The model under review builds one solid part; all positions refer to its coordinate system, in mm. A direction names the side the tool comes from. Round coordinates to 2 decimals unless told otherwise and drop trailing zeros. Write each loop counter-clockwise with the first axis right and the second up, starting at its lowest first coordinate (ties: lowest second). Pieces come first, ordered by that corner, then holes. Notation, with made-up numbers: M 52,72 L 80,72 A9 ccw 80,87 Z; hole C -6,-23.75 d4. An arc over 180 degrees is marked long. Write item = value, one per line. Start each with the question number.
Item 1: Take a section at A-A, the plane x = 0. Give the boundary of the cut face in (y, z) (3 decimals).
Item 2: Tool access review of faces 1 (the cylindrical face through (12.91, 4.83, 15.33)), 2 (the flat face through (-22.225, 5, 2)), 3 (the flat face through (22.225, 5, 2)): name each direction out of +Z, -Z, +X, -X, +Y, -Y from which nothing blocks a thin tool from reaching the whole face with its end or side.
Item 3: For pin 1 Ø25 at (x, z) = (0, 0) entering from +Y; pin 2 Ø3 at (y, z) = (4, -8.5) entering from +X (3 decimals); pin 3 Ø5 at (x, y) = (34.5, 6.5) entering from -Z; pin 4 Ø5 at (y, z) = (4, 9.5) entering from -X (3 decimals), all flat-tipped, find the tip position at first contact; note any pin that passes through.
Item 4: Take a section at B-B, the plane z = 0. Give the boundary of the cut face in (x, y) (3 decimals).
Item 5: To check wall thickness, follow line 1 along X through (y, z) = (3.5, 0) (3 decimals); line 2 along Z through (x, y) = (0, 2.5) (3 decimals); line 3 along Z through (x, y) = (36, 9.25). State the ranges of each line that lie inside material, in increasing order.
Item 6: Take a section at C-C, the plane x = 34. Give the boundary of the cut face in (y, z) (3 decimals), plus the area to 3 significant figures.
Item 7: Take a section at D-D, the plane z = -17.5. Give the boundary of the cut face in (x, y) (3 decimals).
Item 8: The part is to be moulded in two halves that separate along X. For faces 4 (the cylindrical face through (-24.135, 4.829, 29.939)), 5 (the cylindrical face through (8.329, 4.829, -13.065)), 6 (the flat face through (35, 5, 31.75)), say which applies: +X half, -X half, draft (parallel to the pull), parting line (faces both ways), or undercut.
from build123d import *

# Parameters (mm, degrees)
SKETCH1_W             = 44.45
SKETCH1_H             = 60.325
BOSS_EXTRUDE1_DEPTH   = 9.525
SKETCH7_W             = 22.225
SKETCH7_H             = 9.525
BOSS_EXTRUDE3_DEPTH   = 6.35
FILLET1_R             = 6.35
SKETCH8_R             = 2.4892
CUT_EXTRUDE1_DEPTH    = 6.35
CUT_EXTRUDE2_REACH    = 11.525
SKETCH10_R            = 15.494
SKETCH10_R_2          = 1.7272
F_8_32_TAPPED_HOLE2_D = 3.4544


with BuildPart() as part:
    # Sketch1 → Boss-Extrude1 (new body)
    with BuildSketch(Plane(origin=(0, 0, 0), x_dir=(1, 0, 0), z_dir=(0, 1, 0))):
        with Locations((0, -7.9375)):
            Rectangle(SKETCH1_W, SKETCH1_H)
    extrude(amount=BOSS_EXTRUDE1_DEPTH)

    # Sketch7 → Boss-Extrude3 (add)
    with BuildSketch(Plane.XY.offset(38.1)):
        with Locations((-33.3375, 4.7625)):
            Rectangle(SKETCH7_W, SKETCH7_H)
        with Locations((33.3375, 4.7625)):
            Rectangle(SKETCH7_W, SKETCH7_H)
    extrude(amount=-BOSS_EXTRUDE3_DEPTH)

    # Fillet1
    fillet1_edges = [part.edges().sort_by_distance(p)[0] for p in [
        (-22.225, 4.7625, 31.75),
        (22.225, 4.7625, 31.75),
    ]]
    fillet(fillet1_edges, radius=FILLET1_R)

    # Sketch8 → Cut-Extrude1 (cut)
    with BuildSketch(Plane.XY.offset(38.1)):
        with Locations((-38.1, 4.7625)):
            Circle(SKETCH8_R)
        with Locations((38.1, 4.7625)):
            Circle(SKETCH8_R)
    extrude(amount=-CUT_EXTRUDE1_DEPTH, mode=Mode.SUBTRACT)

    # Sketch10 → Cut-Extrude2 (cut, up to next)
    with BuildSketch(Plane(origin=(0, 9.525, 0), x_dir=(1, 0, 0), z_dir=(0, 1, 0)), mode=Mode.PRIVATE) as cut_extrude2_sk1:
        Circle(SKETCH10_R)
    cut_extrude2_tool1 = extrude(cut_extrude2_sk1.sketch, amount=-CUT_EXTRUDE2_REACH, mode=Mode.PRIVATE) & part.part
    add(cut_extrude2_tool1.solids().sort_by_distance((0, 9.525, 0))[0], mode=Mode.SUBTRACT)
    # Sketch10 → Cut-Extrude2 (cut, up to next)
    with BuildSketch(Plane(origin=(0, 9.525, 0), x_dir=(1, 0, 0), z_dir=(0, 1, 0)), mode=Mode.PRIVATE) as cut_extrude2_sk2:
        with Locations((-14.278607233, 14.278607232)):
            Circle(SKETCH10_R_2)
    cut_extrude2_tool2 = extrude(cut_extrude2_sk2.sketch, amount=-CUT_EXTRUDE2_REACH, mode=Mode.PRIVATE) & part.part
    add(cut_extrude2_tool2.solids().sort_by_distance((-14.278607, 9.525, -14.278607))[0], mode=Mode.SUBTRACT)
    # Sketch10 → Cut-Extrude2 (cut, up to next)
    with BuildSketch(Plane(origin=(0, 9.525, 0), x_dir=(1, 0, 0), z_dir=(0, 1, 0)), mode=Mode.PRIVATE) as cut_extrude2_sk3:
        with Locations((14.278607232, -14.278607232)):
            Circle(SKETCH10_R_2)
    cut_extrude2_tool3 = extrude(cut_extrude2_sk3.sketch, amount=-CUT_EXTRUDE2_REACH, mode=Mode.PRIVATE) & part.part
    add(cut_extrude2_tool3.solids().sort_by_distance((14.278607, 9.525, 14.278607))[0], mode=Mode.SUBTRACT)

    # #8-32 Tapped Hole2 (through all)
    with Locations(Plane(origin=(0, 9.525, 0), x_dir=(1, 0, 0), z_dir=(0, 1, 0))):
        with Locations((-14.278607233, 14.278607232), (14.278607232, -14.278607232)):
            Hole(F_8_32_TAPPED_HOLE2_D / 2)


solid = part.part
Response values:
q1.outline = M 0,-22.225 L 9.525,-22.225 L 9.525,-15.494 L 0,-15.494 Z; M 0,15.494 L 9.525,15.494 L 9.525,38.1 L 0,38.1 Z
q2.face_1 = +Y, -Y
q2.face_2 = -Z, -X, +Y, -Y
q2.face_3 = -Z, +X, +Y, -Y
q3.pin_1 = through
q3.pin_2 = 22.225
q3.pin_3 = 31.75
q3.pin_4 = -22.225
q4.outline = M -22.225,0 L -15.494,0 L -15.494,9.525 L -22.225,9.525 Z; M 15.494,0 L 22.225,0 L 22.225,9.525 L 15.494,9.525 Z
q5.line_1 = -22.225 to -15.494, 15.494 to 22.225
q5.line_2 = -22.225 to -15.494, 15.494 to 38.1
q5.line_3 = 31.75 to 38.1
q6.outline = M 0,31.75 L 9.525,31.75 L 9.525,38.1 L 0,38.1 Z
q6.area = 60.5 mm2
q7.outline = M -22.225,0 L 22.225,0 L 22.225,9.525 L -22.225,9.525 Z
q8.face_4 = -X half
q8.face_5 = undercut
q8.face_6 = draft
